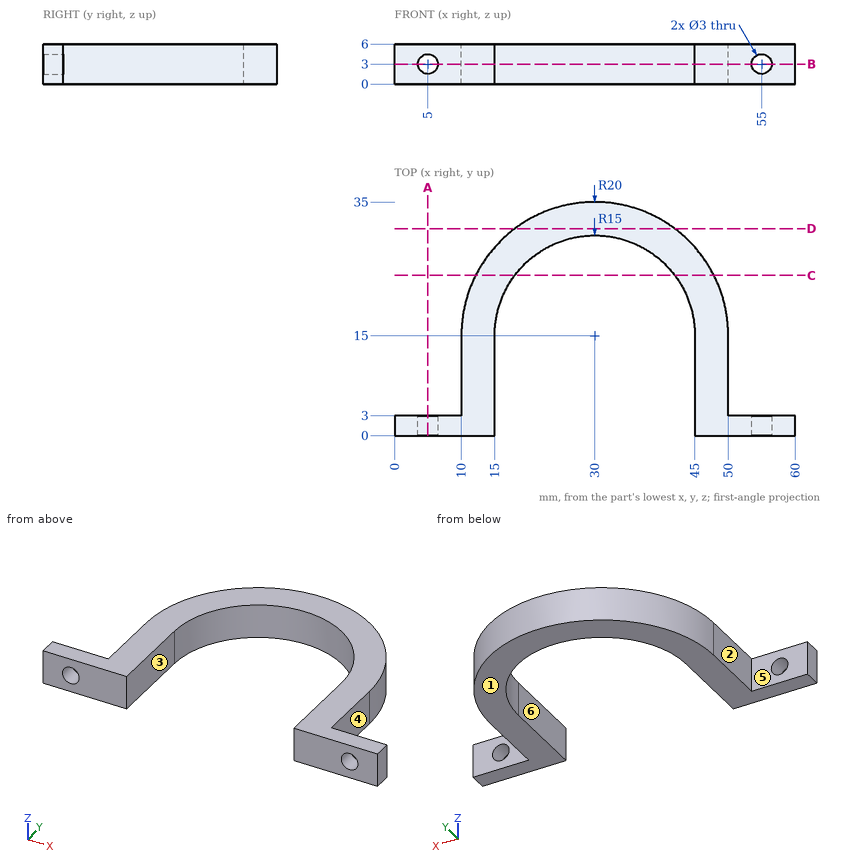
Answer from the drawing. Dimensions are ordinates in mm from the lowest x, y and z of the part. A direction names the side the tool comes from. Coordinates: 2 decimals unless noted, no trailing zeros. Loops run counter-clockwise (first coordinate to the right, second up) from the corner with the lowest first, then second, coordinate; pieces in that order, holes last.
1) For a pull along X with two mould halves and no side action, classify the marked faces 1, 2 and 3 as +X half, -X half, draft (parallel to the pull), parting line (faces both ways), or undercut.
Results:
face 1: draft
face 2: -X half
face 3: undercut
2) Section D-D (y = 31) is taken. Give the vertices of the cut face in (x, z).
Results:
outline: (18, 0) - (42, 0) - (42, 6) - (18, 6) - close
3) Flat-ended cylindrical pins translate along their axes: pin 1 (3 mm diameter, centred on y = 18.5, z = 1, fed in from -X); pin 2 (1.8 mm diameter, centred on x = 4.5, z = 4, fed in from +Y); pin 3 (2 mm diameter, centred on y = 10, z = 3, fed in from +X). Find the tip coordinate at first contact, or state that the pin passes through.
Results:
pin 1: stops at x = 10.1
pin 2: stops at y = 3
pin 3: stops at x = 50
4) Section A-A (x = 5) is taken. Give the vertices of the cut face in (y, z), plus the area to 3 significant figures.
Results:
outline: (0, 0) - (3, 0) - (3, 1.5) - (0, 1.5) - close; (0, 4.5) - (3, 4.5) - (3, 6) - (0, 6) - close
area: 9.00 mm2
5) Consider probe 1 along X at (y, z) = (2.3, 3); probe 2 along X at (y, z) = (4, 4.9); probe 3 along Z at (x, y) = (55, 1.4). Determine where each line is inside the solid, lowest interval first.
Results:
probe 1: x = 0 to 3.5, 6.5 to 15, 45 to 53.5, 56.5 to 60
probe 2: x = 10 to 15, 45 to 50
probe 3: z = 0 to 1.5, 4.5 to 6
6) Section C-C (y = 24) is taken. Give the vertices of the cut face in (x, z).
Results:
outline: (12.14, 0) - (18, 0) - (18, 6) - (12.14, 6) - close; (42, 0) - (47.86, 0) - (47.86, 6) - (42, 6) - close
7) Section B-B (z = 3) is taken. Give the vertices of the cut face in (x, y), plus the area to 3 significant figures.
Results:
outline: (0, 0) - (3.5, 0) - (3.5, 3) - (0, 3) - close; (6.5, 0) - (15, 0) - (15, 15) arc R15 cw to (45, 15) - (45, 0) - (53.5, 0) - (53.5, 3) - (50, 3) - (50, 15) arc R20 ccw to (10, 15) - (10, 3) - (6.5, 3) - close; (56.5, 0) - (60, 0) - (60, 3) - (56.5, 3) - close
area: 467 mm2
8) For the marked faces 4, 5 and 6, determine the directions among +Z, -Z, +X, -X, +Y, -Y from which every point of the face is accessible in a straight line to the end or side of a thin tool.
Results:
face 4: +Z, -Z, +X, +Y
face 5: +Z, -Z, -X, +Y
face 6: +Z, -Z, -Y
